```python
from build123d import *

# Parameters (mm, degrees)
SKETCH1_R           = 4.1
SKETCH1_R_2         = 1.6
BOSS_EXTRUDE1_DEPTH = 5
CHAMFER1_SIZE       = 1.7
CUT_EXTRUDE1_DEPTH  = 3


with BuildPart() as part:
    # Sketch1 → Boss-Extrude1 (new body)
    with BuildSketch(Plane(origin=(0, 0, 0), x_dir=(1, 0, 0), z_dir=(0, 1, 0))):
        with BuildLine():
            Line((-20.432418055, 3.512858569), (-7.567581945, 11.778442321))
            ThreePointArc((-7.567581945, 11.778442321), (0, 14), (7.567581945, 11.778442321))
            Line((7.567581945, 11.778442321), (20.432418055, 3.512858569))
            ThreePointArc((20.432418055, 3.512858569), (22.350852961, 0), (20.432418055, -3.512858569))
            Line((20.432418055, -3.512858569), (7.567581945, -11.778442321))
            ThreePointArc((7.567581945, -11.778442321), (0, -14), (-7.567581945, -11.778442321))
            Line((-7.567581945, -11.778442321), (-20.432418055, -3.512858569))
            ThreePointArc((-20.432418055, -3.512858569), (-22.350852961, 0), (-20.432418055, 3.512858569))
        make_face()
        with Locations(Location((0, 0, 0), (0, 0, 270))):
            Circle(SKETCH1_R, mode=Mode.SUBTRACT)
        with Locations(Location((-18.175426481, 0, 0), (0, 0, 270))):
            Circle(SKETCH1_R_2, mode=Mode.SUBTRACT)
        with Locations(Location((18.175426481, 0, 0), (0, 0, 270))):
            Circle(SKETCH1_R_2, mode=Mode.SUBTRACT)
        with Locations(Location((0, 8, 0), (0, 0, 270))):
            Circle(SKETCH1_R_2, mode=Mode.SUBTRACT)
        with Locations(Location((8, 0, 0), (0, 0, 270))):
            Circle(SKETCH1_R_2, mode=Mode.SUBTRACT)
        with Locations(Location((0, -8, 0), (0, 0, 270))):
            Circle(SKETCH1_R_2, mode=Mode.SUBTRACT)
        with Locations(Location((-8, 0, 0), (0, 0, 270))):
            Circle(SKETCH1_R_2, mode=Mode.SUBTRACT)
    extrude(amount=BOSS_EXTRUDE1_DEPTH)

    # Chamfer1
    chamfer1_edges = [part.edges().sort_by_distance(p)[0] for p in [
        (0, 5, -9.6),
        (8, 5, -1.6),
        (0, 5, 6.4),
        (-8, 5, -1.6),
    ]]
    chamfer(chamfer1_edges, length=CHAMFER1_SIZE)

    # Sketch2 → Cut-Extrude1 (cut)
    with BuildSketch(Plane.XZ):
        Polygon((-15, 0), (-16.58771324, 2.75), (-19.763139721, 2.75), (-21.350852961, 0), (-19.763139721, -2.75), (-16.58771324, -2.75), align=None)
        Polygon((15, 0), (16.58771324, -2.75), (19.763139721, -2.75), (21.350852961, 0), (19.763139721, 2.75), (16.58771324, 2.75), align=None)
    extrude(amount=-CUT_EXTRUDE1_DEPTH, mode=Mode.SUBTRACT)


solid = part.part
```
Design review of the part built by this model. Coordinates are the model's own, in mm. A direction names the side the tool comes from. Coordinates: 2 decimals unless noted, no trailing zeros. Order: outer loops, then holes, each group sorted by start corner. A loop starts at its lowest first (then second) coordinate and runs counter-clockwise, first axis right, second up. Notation, with made-up numbers: (2.5, -22) -> (12.5, -22) arc R36 ccw to (12.5, 16) -> close; hole circle Ø6 at (87, 86). An arc over 180 degrees is marked (long way). One line per item, written item: value. Start each with the question number.
Q1. Tool access review of faces 1 (the flat face through (18, 1, -2.75)), 2 (the cylindrical face through (0.07, 1.63, 6.4)): name each direction out of +Z, -Z, +X, -X, +Y, -Y from which nothing blocks a thin tool from reaching the whole face with its end or side.
Q2. Take a section at B-B, the plane y = 1.05. State the section outline as (x, z) points.
Q3. Take a section at A-A, the plane x = 0. State the section outline as (y, z) points, then the cut area to 3 significant figures.
Q4. For probe 1 along X at (y, z) = (2, 0); probe 2 along X at (y, z) = (1.85, -2.5); probe 3 along Z at (x, y) = (-1.5, 3.6), list the stretches that pass through material, from the lowest coordinate up.
Q5. Take a section at C-C, the plane z = 8. State the section outline as (x, y) points.
Q6. Insertion check: pin 1 Ø1.5 at (x, y) = (-18, 1.5) entering from +Z; pin 2 Ø3.5 at (x, z) = (18.18, 0) entering from -Y; pin 3 Ø0.9 at (x, y) = (19, 2) entering from +Z; pin 4 Ø3 at (x, z) = (8, 0) entering from -Y. Each pin has a flat end and moves straight along its axis. Give the tip position at first contact, or say it passes through.
Q7. Take a section at D-D, the plane x = -8. State the section outline as (y, z) points.
Q8. Mouldability with a two-part tool opening along X and no side actions: class faces 3 (the cylindrical face through (-22.35, 2.46, 0.06)), 4 (the flat face through (14.09, 2.46, 7.59)), 5 (the flat face through (5, 5, -3)), 6 (the conical face through (1.153, 3.406, 6.742)) as pulls with the +X half, pulls with the -X half, needs draft (parallel to the pull), parting line crosses it, or undercut.
Values follow:
1. face 1: -Y
1. face 2: +Y, -Y
2. outline: (-20.43, -3.51) -> (-7.57, -11.78) arc R14 ccw to (7.57, -11.78) -> (20.43, -3.51) arc R4.18 ccw to (20.43, 3.51) -> (7.57, 11.78) arc R14 ccw to (-7.57, 11.78) -> (-20.43, 3.51) arc R4.18 ccw to start; hole (-21.35, 0) -> (-19.76, -2.75) -> (-16.59, -2.75) -> (-15, 0) -> (-16.59, 2.75) -> (-19.76, 2.75) -> close; hole circle Ø3.2 at (-8, 0); hole circle Ø8.2 at (0, 0); hole circle Ø3.2 at (0, -8); hole circle Ø3.2 at (0, 8); hole circle Ø3.2 at (8, 0); hole (15, 0) -> (16.59, -2.75) -> (19.76, -2.75) -> (21.35, 0) -> (19.76, 2.75) -> (16.59, 2.75) -> close
3. outline: (0, -14) -> (5, -14) -> (5, -11.3) -> (3.3, -9.6) -> (0, -9.6) -> close; (0, -6.4) -> (3.3, -6.4) -> (5, -4.7) -> (5, -4.1) -> (0, -4.1) -> close; (0, 4.1) -> (5, 4.1) -> (5, 4.7) -> (3.3, 6.4) -> (0, 6.4) -> close; (0, 9.6) -> (3.3, 9.6) -> (5, 11.3) -> (5, 14) -> (0, 14) -> close
3. area: 61.2 mm2
4. probe 1: x = -22.35 to -21.35, -15 to -9.6, -6.4 to -4.1, 4.1 to 6.4, 9.6 to 15, 21.35 to 22.35
4. probe 2: x = -21.52 to -19.91, -16.44 to -3.25, 3.25 to 16.44, 19.91 to 21.52
4. probe 3: z = -13.92 to -9.17, -6.83 to -3.82, 3.82 to 6.83, 9.17 to 13.92
5. outline: (-13.45, 0) -> (-1.6, 0) -> (-1.6, 3.3) -> (-3.3, 5) -> (-13.45, 5) -> close; (1.6, 0) -> (13.45, 0) -> (13.45, 5) -> (3.3, 5) -> (1.6, 3.3) -> close
6. pin 1: stops at z = 5.56
6. pin 2: stops at y = 3
6. pin 3: stops at z = 4.72
6. pin 4: passes through
7. outline: (0, -11.5) -> (5, -11.5) -> (5, -3.3) -> (3.3, -1.6) -> (0, -1.6) -> close; (0, 1.6) -> (3.3, 1.6) -> (5, 3.3) -> (5, 11.5) -> (0, 11.5) -> close
8. face 3: pulls with the -X half
8. face 4: pulls with the +X half
8. face 5: needs draft
8. face 6: undercut
